Here's how the part is built. I have some questions about the finished solid (model axes, mm). Face numbers are marked on the shaded views. A direction names the side the tool comes from. Round coordinates to 2 decimals unless told otherwise and drop trailing zeros. Write each loop counter-clockwise with the first axis right and the second up, starting at its lowest first coordinate (ties: lowest second). Pieces come first, ordered by that corner, then holes. Notation, with made-up numbers: (68.25, 50.5) -> (110.25, 50.5) arc R20 ccw to (110.25, 85.5) -> close; hole circle Ø3 at (31, 47.5). An arc over 180 degrees is marked (long way). Answer as CSV lines item,"result".
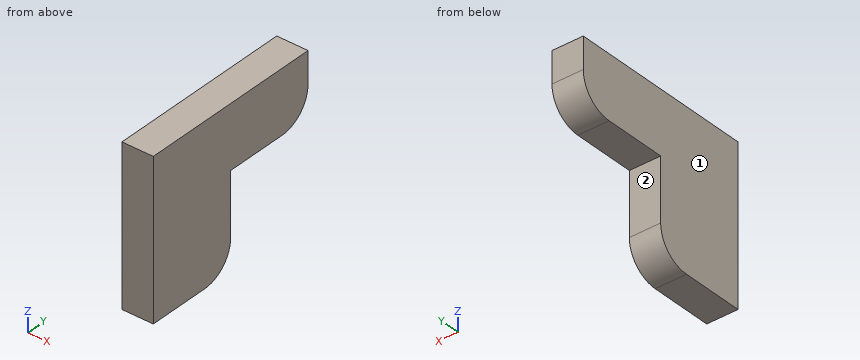
from build123d import *

# Parameters (mm, degrees)
F0_W     = 10
F0_H     = 40
F0_H_2   = 10
F0_W_2   = 30
F1_DEPTH = 10


with BuildPart() as f1:
    # F0 (on Right) → F1 (new body)
    with BuildSketch(Plane.YZ):
        with Locations((5, 20)):
            Rectangle(F0_W, F0_H)
        with Locations((55, 45)):
            Rectangle(F0_W, F0_H_2)
        Polygon((0, 50), (0, 40), (10, 40), (20, 40), (20, 50), align=None)
        with Locations((35, 45)):
            Rectangle(F0_W_2, F0_H_2)
        with BuildLine():
            Line((10, 40), (10, 0))
            Line((10, 0), (20, 0))
            ThreePointArc((20, 0), (27.071068, 2.928932), (30, 10))
            Line((30, 10), (30, 30))
            Line((30, 30), (40, 30))
            Line((40, 30), (50, 30))
            ThreePointArc((50, 30), (57.071068, 32.928932), (60, 40))
            Line((60, 40), (50, 40))
            Line((50, 40), (20, 40))
            Line((20, 40), (10, 40))
        make_face()
    extrude(amount=F1_DEPTH)


solid = f1.part
Item 1: Will these pins go through, and if not, where does the flat tip stop? pin 1 (3 mm diameter, centred on x = 4.5, z = 20, fed in from +Y); pin 2 (5 mm diameter, centred on x = 7, y = 41, fed in from -Z).
Results found:
pin 1,"stops at y = 30"
pin 2,"stops at z = 30"
Item 2: I need wall thicknesses on L1, parallel to Z at x = 2.75, y = 33; L2, parallel to Y at x = 9, z = 29.5; L3, parallel to Y at x = 9.5, z = 32. Which ranges of each line are inside material? Lowest first, please.
Results found:
L1,"z = 30 to 50"
L2,"y = 0 to 30"
L3,"y = 0 to 56"
Item 3: For the marked faces 1 and 2, which set-ups out of +Z, -Z, +X, -X, +Y, -Y let a thin tool reach every point of the face, with its end or its side?
Results found:
face 1,"+Z, -Z, -X, +Y, -Y"
face 2,"-Z, +X, -X, +Y"
Item 4: Suppose I cut it at B-B, the plane z = 4. List the corners of the cut face in (x, y) for me.
Results found:
outline,"(0, 0) -> (10, 0) -> (10, 28) -> (0, 28) -> close"
Item 5: Suppose I cut it at C-C, the plane y = 48.5. List the corners of the cut face in (x, z) for me, then the cut area to 3 significant figures.
Results found:
outline,"(0, 30) -> (10, 30) -> (10, 50) -> (0, 50) -> close"
area,"200 mm²"
Item 6: Suppose I cut it at A-A, the plane x = 7. List the corners of the cut face in (y, z) for me.
Results found:
outline,"(0, 0) -> (20, 0) arc R10 ccw to (30, 10) -> (30, 30) -> (50, 30) arc R10 ccw to (60, 40) -> (60, 50) -> (0, 50) -> close"
